```python
from build123d import *

# Parameters (mm, degrees)
SKETCH2_W                  = 21.2
SKETCH2_H                  = 10
F_6_0_204_DIAMETER_HOLE1_D = 5.1816
CUT_EXTRUDE1_DEPTH         = 11
CIRPATTERN1_COUNT          = 4
FILLET1_R                  = 5


with BuildPart() as part:
    # Sketch2 → Revolve1 (revolve)
    with BuildSketch(Plane(origin=(0, 0, 0), x_dir=(0, 0, -1), z_dir=(1, 0, 0))):
        with Locations((-65.6, 5)):
            Rectangle(SKETCH2_W, SKETCH2_H)
    revolve(axis=Axis((0, 3.678923398, 0), (0, 1, 0)))

    # #6 (0.204) Diameter Hole1 (through all)
    with Locations(Plane(origin=(0, 0, 0), x_dir=(-1, 0, 0), z_dir=(0, -1, 0))):
        with Locations((36.390872965, 48.461940777)):
            f_6_0_204_diameter_hole1 = Hole(F_6_0_204_DIAMETER_HOLE1_D / 2)

    # Sketch14 → Cut-Extrude1 (cut, through all)
    with BuildSketch(Plane.XZ):
        with BuildLine():
            Line((-33.070789849, -38.070789849), (-47.783894042, -52.783894042))
            ThreePointArc((-47.783894042, -52.783894042), (-70.683932228, -8.55696937), (-58.998941132, 39.856805508))
            Line((-58.998941132, 39.856805508), (-55.533008589, 36.390872965))
            Line((-55.533008589, 36.390872965), (-48.461940777, 29.319805153))
            Line((-48.461940777, 29.319805153), (-41.390872965, 36.390872965))
            Line((-41.390872965, 36.390872965), (-38.070789849, 33.070789849))
            ThreePointArc((-38.070789849, 33.070789849), (-50.304693428, -3.535533906), (-33.070789849, -38.070789849))
        make_face()
    cut_extrude1 = extrude(amount=-CUT_EXTRUDE1_DEPTH, mode=Mode.SUBTRACT)

    # CirPattern1: #6 (0.204) Diameter Hole1, Cut-Extrude1 ×4 about axis
    cirpattern1_axis = Axis((0, 0, 0), (0, 1, 0))
    for i in range(1, CIRPATTERN1_COUNT):
        add(f_6_0_204_diameter_hole1.rotate(cirpattern1_axis, i * 360 / CIRPATTERN1_COUNT), mode=Mode.SUBTRACT)
        add(cut_extrude1.rotate(cirpattern1_axis, i * 360 / CIRPATTERN1_COUNT), mode=Mode.SUBTRACT)

    # Fillet1
    fillet1_edges = [part.edges().sort_by_distance(p)[0] for p in [
        (-47.783894042, 5, -52.783894042),
        (-58.998941132, 5, 39.856805508),
        (-52.783894042, 5, 47.783894042),
        (39.856805508, 5, 58.998941132),
        (47.783894042, 5, 52.783894042),
        (58.998941132, 5, -39.856805508),
        (52.783894042, 5, -47.783894042),
        (-39.856805508, 5, -58.998941132),
    ]]
    fillet(fillet1_edges, radius=FILLET1_R)


solid = part.part
```
For this review, take the finished solid that the model builds, in its own axes (mm). Round coordinates to 2 decimals unless told otherwise and drop trailing zeros. Write each loop counter-clockwise with the first axis right and the second up, starting at its lowest first coordinate (ties: lowest second). Pieces come first, ordered by that corner, then holes. Notation, with made-up numbers: M 47,37 L 74,37 A23 cw 74,62 Z; hole C -29.75,-31.75 d8. An arc over 180 degrees is marked long. One line per item, written item: value. Start each with the question number.
(1) We need section A-A (x = 0). Give the boundary of the cut face in (y, z).
(2) Insertion check: pin 1 (4 mm diameter, centred on y = 6, z = 47, fed in from +X); pin 2 (3 mm diameter, centred on x = 20, y = 9, fed in from +Z); pin 3 (3 mm diameter, centred on x = 48.46, z = -36.39, fed in from -Y); pin 4 (5 mm diameter, centred on y = 5.5, z = 33.5, fed in from -X). Each pin has a flat end and moves straight along its axis. Give the tip position at first contact, or say it passes through.
(3) We need section C-C (y = 6.75). Count the separate pieces of the cut face and the enclosed holes in it, and give its area (3 significant figures).
(4) The part is to be moulded in two halves that separate along Z. For faces 1 (the cylindrical face through (-46.367, 5.07, -60.47)), 2 (the flat face through (46, 0, -34)), 3 (the cylindrical face through (-70.506, 4.93, -9.913)), say which applies: released by +Z, released by -Z, zero draft, split by the parting line, or undercut.
(5) Wall thickness on line 1 (Z direction, x = 30.5, y = 5); line 2 (X direction, y = 2.75, z = -29.5); line 3 (X direction, y = 3, z = 1): over which ranges is each line inside the solid? List them lowest first.
(6) We need section B-B (z = 0). Give the boundary of the cut face in (x, y).
Result:
1. outline: M 0,-76.2 L 10,-76.2 L 10,-71.2 L 0,-71.2 Z; M 0,71.2 L 10,71.2 L 10,76.2 L 0,76.2 Z
2. pin 1: x = 61.49
2. pin 2: z = 73.92
2. pin 3: through
2. pin 4: x = -69.61
3. separate pieces: 1
3. enclosed holes: 5
3. area: 2,920 mm²
4. face 1: split by the parting line
4. face 2: zero draft
4. face 3: undercut
5. line 1: -69.83 to -64.34, 47.28 to 49.64, 64.34 to 69.83
5. line 2: -70.26 to -64.8, 48.28 to 48.64, 64.8 to 70.26
5. line 3: -76.19 to -71.19, 71.19 to 76.19
6. outline: M -76.2,0 L -71.2,0 L -71.2,10 L -76.2,10 Z; M 71.2,0 L 76.2,0 L 76.2,10 L 71.2,10 Z
